Build history of the part. All positions in model axes, mm. A direction names the side the tool comes from. Coordinates: 2 decimals unless noted, no trailing zeros. Loops run counter-clockwise (first coordinate to the right, second up) from the corner with the lowest first, then second, coordinate; pieces in that order, holes last.
Item 1: Drill centre lines: line 1 along X through (y, z) = (2.25, -5); line 2 along X through (y, z) = (3, -5); line 3 along Y through (x, z) = (17, -11.25). Where is each one in solid material? Low to high.
Item 2: Mould opens along Y. For faces 1 (the face through (37.564, 0.07, -14.917)), 2 (the face through (30.037, 7.178, -13.792)), 3 (the face through (-28.799, -7.178, -4.999)), 4 (the face through (26.035, -1.724, -13.194)) say: released by +Y, released by -Y, zero draft, split by the parting line, or undercut.
Item 3: Cut at A-A (y = -3.5). List the corners of the cut face in (x, z), and give its area (3 significant figures).
Item 4: 3-axis set-ups, long thin cutter, end or side, ignore diameter. For faces 5 (the face through (23.478, 0, -4)), 6 (the face through (-24.444, -1.352, -5.65)): which of +Z, -Z, +X, -X, +Y, -Y reach the whole face in a straight line?
Item 5: Cut at B-B (z = -5). Count the separate pieces of the cut face and the enclosed holes in it, and give its area (3 significant figures).
Item 6: Cut at C-C (y = 3.75). List the corners of the cut face in (x, z).
Item 7: Cut at D-D (x = -13.5). List the corners of the cut face in (y, z).
Item 8: Flat gauge pins, fed straight in: pin 1 (1 mm diameter, centred on x = 14.5, z = -13, fed in from -Y); pin 2 (6 mm diameter, centred on y = 0, z = -3, fed in from +X); pin 3 (1 mm diameter, centred on y = 3, z = -1, fed in from -X). Where does each tip first touch, or does it go through?
from build123d import *

# Parameters (mm, degrees)
EXTRUDE_2_DEPTH     = 5
SKETCH_4_R          = 4.5
EXTRUDE_3_DEPTH     = 10
EXTRUDE_4_DEPTH     = 5
CUT_EXTRUDE_1_DEPTH = 5
EXTRUDE_5_DEPTH     = 5
CUT_EXTRUDE_2_DEPTH = 5
SKETCH_9_R          = 2.1
CUT_EXTRUDE_3_DEPTH = 5


with BuildPart() as part:
    # Sketch 3 → Extrude 2 (new, symmetric)
    with BuildSketch(Plane(origin=(0, 0, 0), x_dir=(1, 0, 0), z_dir=(0, 1, 0))):
        Polygon((-22, 0), (-22, 11), (22, 17.575844059), (22, 0), align=None)
    extrude(amount=EXTRUDE_2_DEPTH, both=True)

    # Sketch 4 → Extrude 3 (add)
    # profile 1 of 2: a face of its own
    with BuildSketch(Plane(origin=(-2.08869206, 0, -13.97576491), x_dir=(-0.9890158633619178, 0, 0.1478094111296043), z_dir=(-0.1478094111296043, 0, -0.9890158633619178))):
        with BuildLine():
            Line((-24.356224154, -5), (-24.356224154, 5))
            ThreePointArc((-24.356224154, 5), (-31.856224154, 7.178409582), (-39.356224154, 5))
            Line((-39.356224154, 5), (-39.356224154, -5))
            ThreePointArc((-39.356224154, -5), (-31.856224154, -7.178409582), (-24.356224154, -5))
        make_face()
        with Locations((-31.856224154, 0)):
            Circle(SKETCH_4_R, mode=Mode.SUBTRACT)
    # profile 2 of 2: a face of its own
    with BuildSketch(Plane(origin=(-2.08869206, 0, -13.97576491), x_dir=(-0.9890158633619178, 0, 0.1478094111296043), z_dir=(-0.1478094111296043, 0, -0.9890158633619178))):
        with BuildLine():
            Line((35.132445472, 5), (35.132445472, -5))
            ThreePointArc((35.132445472, -5), (27.632445472, -7.178409582), (20.132445472, -5))
            Line((20.132445472, -5), (20.132445472, 5))
            ThreePointArc((20.132445472, 5), (27.632445472, 7.178409582), (35.132445472, 5))
        make_face()
        with Locations(Location((27.632445472, 0, 0), (0, 0, 180))):
            Circle(SKETCH_4_R, mode=Mode.SUBTRACT)
    extrude(amount=-EXTRUDE_3_DEPTH)


with BuildPart() as extrude_3_piece_1:
    # of the separate pieces the step leaves, piece 1, a body of its own (extrude_3_pieces)
    add(part.part.solids().sort_by_distance((-22, -5, 0))[0])



with BuildPart() as extrude_3_piece_2:
    # of the separate pieces the step leaves, piece 2, a body of its own (extrude_3_pieces)
    add(part.part.solids().sort_by_distance((23.478094111, -5, -7.685685426))[0])


with BuildPart() as extrude_3_piece_1_1:
    add(extrude_3_piece_1.part)

    add(extrude_3_piece_2.part)  # Extrude 4 merges Extrude 3 piece 2
    # Sketch 5 → Extrude 4 (add, symmetric)
    with BuildSketch(Plane(origin=(0, 0, 0), x_dir=(1, 0, 0), z_dir=(0, 1, 0))):
        Polygon((23.478094111, 7.685685426), (22, 7.464782781), (22, 17.575844059), align=None)
    extrude(amount=EXTRUDE_4_DEPTH, both=True)

    # Sketch 6 → Cut-Extrude 1 (cut, symmetric)
    with BuildSketch(Plane(origin=(0, 0, 0), x_dir=(1, 0, 0), z_dir=(0, 1, 0))):
        Polygon((-22, 0), (-22, 0.888938721), (-20.521905889, 1.109841366), (-20.356038985, 0), align=None)
    extrude(amount=CUT_EXTRUDE_1_DEPTH, both=True, mode=Mode.SUBTRACT)

    # Sketch 7 → Extrude 5 (add, symmetric)
    with BuildSketch(Plane(origin=(0, 0, 0), x_dir=(1, 0, 0), z_dir=(0, 1, 0))):
        Polygon((22, 0), (24.626727494, 0), (23.478094111, 7.685685426), (22, 7.464782781), align=None)
    extrude(amount=EXTRUDE_5_DEPTH, both=True)

    # Sketch 8 → Cut-Extrude 2 (cut, symmetric)
    with BuildSketch(Plane(origin=(0, 0, 0), x_dir=(1, 0, 0), z_dir=(0, 1, 0))):
        Polygon((23.478094111, 0), (23.478094111, 7.685685426), (24.626727494, 0), align=None)
    extrude(amount=CUT_EXTRUDE_2_DEPTH, both=True, mode=Mode.SUBTRACT)

    # Sketch 9 → Cut-Extrude 3 (cut, symmetric)
    with BuildSketch(Plane(origin=(0, 0, 0), x_dir=(1, 0, 0), z_dir=(0, 1, 0))):
        with Locations(Location((9.478094111, 5, 0), (0, 0, 270))):
            Circle(SKETCH_9_R)
        with Locations(Location((-6.521905889, 5, 0), (0, 0, 270))):
            Circle(SKETCH_9_R)
    extrude(amount=CUT_EXTRUDE_3_DEPTH, both=True, mode=Mode.SUBTRACT)


solid = extrude_3_piece_1_1.part
Filled sheet:
1. line 1: x = -36.27 to -32.63, -24.75 to -8.62, -4.42 to 7.38, 11.58 to 23.48
1. line 2: x = -36.27 to -32.08, -25.3 to -8.62, -4.42 to 7.38, 11.58 to 23.48
1. line 3: y = -5 to 5
2. face 1: zero draft
2. face 2: released by +Y
2. face 3: released by -Y
2. face 4: undercut
3. outline: (-36.84, -8.78) - (-32.21, -9.47) - (-30.74, 0.42) - (-35.36, 1.11) - close; (-26.62, -10.31) - (26.62, -18.27) - (28.1, -8.38) - (23.48, -7.69) - (23.48, 0) - (-20.36, 0) - (-20.52, -1.11) - (-25.14, -0.42) - close; (32.21, -19.1) - (36.84, -19.79) - (38.31, -9.9) - (33.69, -9.21) - close; hole circle Ø4.2 at (-6.52, -5); hole circle Ø4.2 at (9.48, -5)
3. area: 797 mm2
4. face 5: +Z, +X, +Y, -Y
4. face 6: none
5. separate pieces: 3
5. enclosed holes: 1
5. area: 494 mm2
6. outline: (-36.84, -8.78) - (-31.88, -9.52) - (-30.4, 0.37) - (-35.36, 1.11) - close; (-26.96, -10.26) - (26.96, -18.32) - (28.44, -8.43) - (23.48, -7.69) - (23.48, 0) - (-20.36, 0) - (-20.52, -1.11) - (-25.48, -0.37) - close; (31.88, -19.05) - (36.84, -19.79) - (38.31, -9.9) - (33.36, -9.16) - close; hole circle Ø4.2 at (-6.52, -5); hole circle Ø4.2 at (9.48, -5)
7. outline: (-5, -12.27) - (5, -12.27) - (5, 0) - (-5, 0) - close
8. pin 1: stops at y = -5
8. pin 2: stops at x = 23.48
8. pin 3: stops at x = -35.75
